Part print with two shaded views. Sizes in mm from the minimum x, y, z corner. A direction names the side the tool comes from. Round coordinates to 2 decimals unless told otherwise and drop trailing zeros. Loops run counter-clockwise (first coordinate to the right, second up) from the corner with the lowest first, then second, coordinate; pieces in that order, holes last. Notation, with made-up numbers: M 40,-9.5 L 52,-9.5 A23 cw 52,26.5 Z; hole C 66,10.5 d1. An arc over 180 degrees is marked long. Use a Markdown table: item, result. Add a question column.
Item 1: Saw through at B-B on z = 5.35. Write the cut outline in (x, y) (1 decimal), then the cut area to 3 significant figures.
Item 2: Wall check: L1, parallel to X at y = 6, z = 5.5 (1 decimal); L2, parallel to Y at x = 12, z = 1.75; L3, parallel to Y at x = 4, z = 5.2. Give the ranges that are in metal, low to high. Write a range as from..to.
Item 3: Saw through at A-A on x = 20. Write the cut outline in (y, z).
Item 4: Tool access for the marked faces 1 and 2: list every direction of +Z, -Z, +X, -X, +Y, -Y with a clear straight run to the whole face (end or side of a thin tool).
Item 5: Saw through at D-D on z = 1.3. Write the cut outline in (x, y).
Item 6: Saw through at C-C on y = 5.5. Write the cut outline in (x, z) (1 decimal).
Item 7: Two-plate mould, pull along Y, no slides. Class the marked faces 3, 4 and 5: +Y half, -Y half, draft (parallel to the pull), parting line (faces both ways), or undercut.
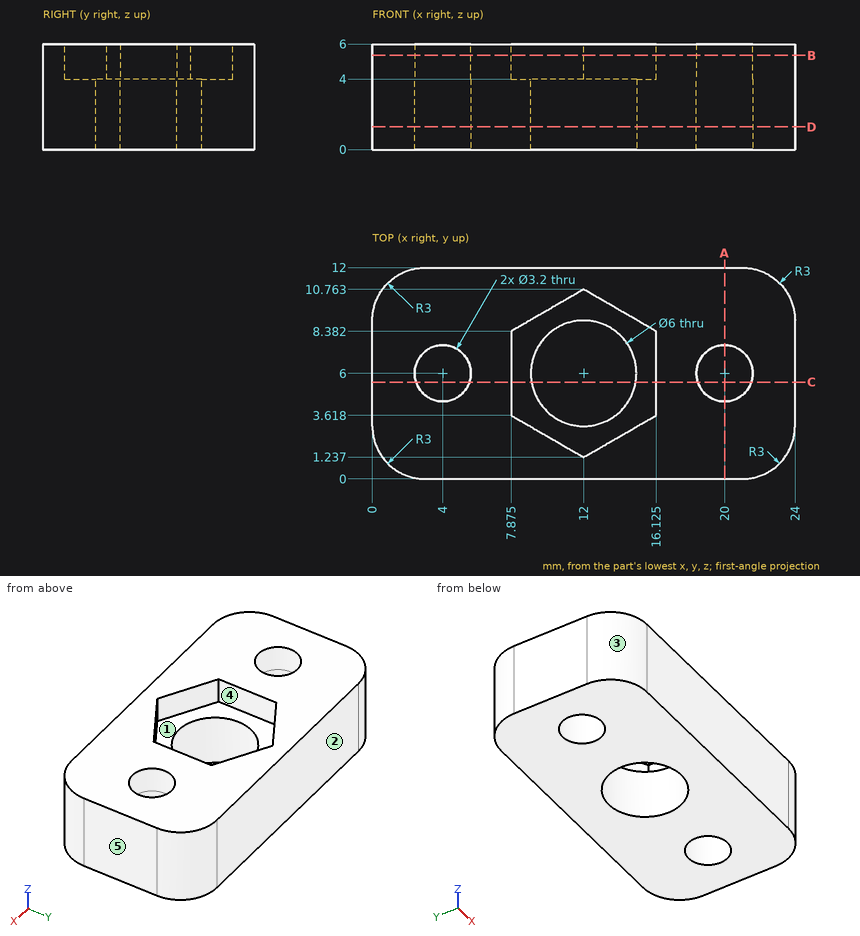
Entries:
| question | item | result |
|---|---|---|
| 1 | outline | M 0,3 A3 ccw 3,0 L 21,0 A3 ccw 24,3 L 24,9 A3 ccw 21,12 L 3,12 A3 ccw 0,9 Z; hole C 4,6 d3.2; hole M 7.9,3.6 L 12,1.2 L 16.1,3.6 L 16.1,8.4 L 12,10.8 L 7.9,8.4 Z; hole C 20,6 d3.2 |
| 1 | area | 205 mm2 |
| 2 | L1 | 0..2.4, 5.6..7.9, 16.1..18.4, 21.6..24 |
| 2 | L2 | 0..3, 9..12 |
| 2 | L3 | 0..4.4, 7.6..12 |
| 3 | outline | M 0,0 L 4.4,0 L 4.4,6 L 0,6 Z; M 7.6,0 L 12,0 L 12,6 L 7.6,6 Z |
| 4 | face 1 | +Z |
| 4 | face 2 | +Z, -Z, +X, -X, +Y |
| 5 | outline | M 0,3 A3 ccw 3,0 L 21,0 A3 ccw 24,3 L 24,9 A3 ccw 21,12 L 3,12 A3 ccw 0,9 Z; hole C 4,6 d3.2; hole C 12,6 d6; hole C 20,6 d3.2 |
| 6 | outline | M 0,0 L 2.5,0 L 2.5,6 L 0,6 Z; M 5.5,0 L 9,0 L 9,4 L 7.9,4 L 7.9,6 L 5.5,6 Z; M 15,0 L 18.5,0 L 18.5,6 L 16.1,6 L 16.1,4 L 15,4 Z; M 21.5,0 L 24,0 L 24,6 L 21.5,6 Z |
| 7 | face 3 | -Y half |
| 7 | face 4 | undercut |
| 7 | face 5 | draft |
